from build123d import *

# Parameters (mm, degrees)
SKETCH1_W           = 381
SKETCH1_H           = 177.8
BOSS_EXTRUDE1_DEPTH = 6.35
CUT_EXTRUDE1_DEPTH  = 421.492761531
CUT_EXTRUDE2_DEPTH  = 421.492761531
LPATTERN1_COUNT     = 5
LPATTERN1_PITCH     = 82.55
SKETCH7_R           = 2.1
CUT_EXTRUDE3_DEPTH  = 421.492761531
CUT_EXTRUDE4_DEPTH  = 421.492761531
LPATTERN3_COUNT     = 2
LPATTERN3_PITCH     = 63.5
CUT_EXTRUDE5_DEPTH  = 421.492761531


with BuildPart() as part:
    # Sketch1 → Boss-Extrude1 (new body)
    with BuildSketch(Plane.XY):
        with Locations((190.5, 88.9)):
            Rectangle(SKETCH1_W, SKETCH1_H)
    extrude(amount=BOSS_EXTRUDE1_DEPTH)

    # Sketch2 → Cut-Extrude1 (cut, through all)
    with BuildSketch(Plane.XY.offset(6.35)):
        with BuildLine():
            Line((12.7, 46.55), (50.8, 46.55))
            ThreePointArc((50.8, 46.55), (52.9, 44.45), (50.8, 42.35))
            Line((50.8, 42.35), (12.7, 42.35))
            ThreePointArc((12.7, 42.35), (10.6, 44.45), (12.7, 46.55))
        make_face()
    extrude(amount=-CUT_EXTRUDE1_DEPTH, mode=Mode.SUBTRACT)

    # Sketch6 → Cut-Extrude2 (cut, through all)
    with BuildSketch(Plane.XY.offset(6.35)):
        Polygon((15.875, 0), (34.925, 0), (34.925, 6.35), (27.94, 6.35), (27.94, 7.874), (30.226, 7.874), (30.226, 11.176), (27.94, 11.176), (27.94, 12.7), (22.86, 12.7), (22.86, 11.176), (20.574, 11.176), (20.574, 7.874), (22.86, 7.874), (22.86, 6.35), (15.875, 6.35), align=None)
    cut_extrude2 = extrude(amount=-CUT_EXTRUDE2_DEPTH, mode=Mode.SUBTRACT)

    # LPattern1: Cut-Extrude2 ×5
    with Locations(*[(i * LPATTERN1_PITCH, 0, 0) for i in range(1, LPATTERN1_COUNT)]):
        add(cut_extrude2, mode=Mode.SUBTRACT)

    # Sketch7 → Cut-Extrude3 (cut, through all)
    with BuildSketch(Plane.XY.offset(6.35)):
        with Locations((355.6, 44.45)):
            Circle(SKETCH7_R)
    extrude(amount=-CUT_EXTRUDE3_DEPTH, mode=Mode.SUBTRACT)

    # Sketch8 → Cut-Extrude4 (cut, through all)
    with BuildSketch(Plane.XY.offset(6.35)):
        Polygon((0, 161.925), (0, 142.875), (6.35, 142.875), (6.35, 149.86), (7.874, 149.86), (7.874, 147.574), (11.176, 147.574), (11.176, 149.86), (12.7, 149.86), (12.7, 154.94), (11.176, 154.94), (11.176, 157.226), (7.874, 157.226), (7.874, 154.94), (6.35, 154.94), (6.35, 161.925), align=None)
    cut_extrude4 = extrude(amount=-CUT_EXTRUDE4_DEPTH, mode=Mode.SUBTRACT)

    # LPattern3: Cut-Extrude4 ×2
    with Locations(*[(0, -i * LPATTERN3_PITCH, 0) for i in range(1, LPATTERN3_COUNT)]):
        add(cut_extrude4, mode=Mode.SUBTRACT)

    # Sketch9 → Cut-Extrude5 (cut, through all)
    with BuildSketch(Plane.XY.offset(6.35)):
        Polygon((0, 34.925), (0, 15.875), (6.35, 15.875), (6.35, 22.86), (7.874, 22.86), (7.874, 20.574), (11.176, 20.574), (11.176, 22.86), (12.7, 22.86), (12.7, 27.94), (11.176, 27.94), (11.176, 30.226), (7.874, 30.226), (7.874, 27.94), (6.35, 27.94), (6.35, 34.925), align=None)
    cut_extrude5 = extrude(amount=-CUT_EXTRUDE5_DEPTH, mode=Mode.SUBTRACT)

    # Mirror2: Cut-Extrude5 across plane
    add(cut_extrude5.mirror(Plane.ZY.offset(-190.5)), mode=Mode.SUBTRACT)


solid = part.part
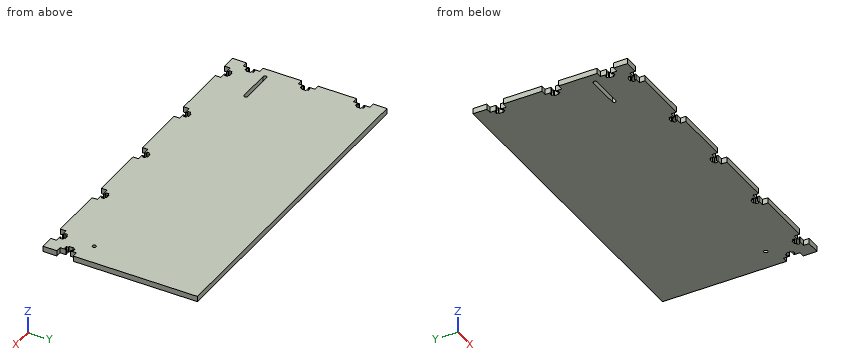
CAD build for the part. Positions are in the model's coordinates, mm. Coordinates: 2 decimals unless noted, no trailing zeros. Answer as a JSON object with one key per item and string values. Group by question number.
1) Saw through at A-A (z = 2.75). Give the number of separate pieces and of enclosed holes in the cut face, plus the area to 3 significant figures.
2) Pin check, flat tip, straight feed: pin 1 Ø1.1 at (y, z) = (148.5, 2.5) entering from -X. Stop position of the tip, or through.
3) Wall check: line 1 (X direction, y = 8, z = 5.25); line 2 (Y direction, x = 355.6, z = 2.25); line 3 (Y direction, x = 105, z = 4.5). Give the ranges that are in metal, low to high. Write a range as from..to.
Values follow:
{
 "1": {"separate pieces": "1", "enclosed holes": "2", "area": "66,000 mm2"},
 "2": {"pin 1": "stops at x = 6.35"},
 "3": {"line 1": "x = 0..20.57, 30.23..103.12, 112.78..185.67, 195.33..268.22, 277.88..350.77, 360.43..381", "line 2": "y = 12.7..42.35, 46.55..177.8", "line 3": "y = 6.35..7.87, 11.18..177.8"}
}
